```python
from build123d import *

# Parameters (mm, degrees)
SKETCH_1_R      = 7
SKETCH_1_R_2    = 4
EXTRUDE_1_DEPTH = 10
SKETCH_2_R      = 4
SKETCH_2_R_2    = 2.2
EXTRUDE_2_DEPTH = 7
CHAMFER_1_SIZE  = 1
CHAMFER_2_SIZE  = 0.5
CHAMFER_3_SIZE  = 0.5


with BuildPart() as part:
    # 草图1 → 凸台-拉伸1 (new body)
    with BuildSketch(Plane.XY):
        with Locations((42.877900702, -281.152618372)):
            Circle(SKETCH_1_R)
        with Locations((42.877900702, -281.152618372)):
            Circle(SKETCH_1_R_2, mode=Mode.SUBTRACT)
    extrude(amount=EXTRUDE_1_DEPTH)

    # 草图2 → 凸台-拉伸2 (add)
    with BuildSketch(Plane.XY.offset(-3)):
        with Locations((42.877900702, -281.152618372)):
            Circle(SKETCH_2_R)
        with Locations((42.877900702, -281.152618372)):
            Circle(SKETCH_2_R_2, mode=Mode.SUBTRACT)
    extrude(amount=EXTRUDE_2_DEPTH)

    # 倒角1
    chamfer_1_edges = [part.edges().sort_by_distance(p)[0] for p in [
        (35.877900702, -281.152618372, 0),
        (35.877900702, -281.152618372, 10),
    ]]
    chamfer(chamfer_1_edges, length=CHAMFER_1_SIZE)

    # 倒角2
    chamfer_2_edges = [part.edges().sort_by_distance(p)[0] for p in [
        (38.877900702, -281.152618372, -3),
    ]]
    chamfer(chamfer_2_edges, length=CHAMFER_2_SIZE)

    # 倒角3
    chamfer_3_edges = [part.edges().sort_by_distance(p)[0] for p in [
        (38.877900702, -281.152618372, 10),
    ]]
    chamfer(chamfer_3_edges, length=CHAMFER_3_SIZE)


solid = part.part
```
Work out the finished part from the listing and answer in its coordinate system (mm). A direction names the side the tool comes from. Coordinates: 2 decimals unless noted, no trailing zeros. Write each loop counter-clockwise with the first axis right and the second up, starting at its lowest first coordinate (ties: lowest second). Pieces come first, ordered by that corner, then holes.
Q1. Find the intervals of material crossed by line 1 (X direction, y = -281.75, z = 7.25); line 2 (X direction, y = -280.5, z = -2); line 3 (Y direction, x = 43.75, z = 5.5), in increasing order.
Q2. A cutting plane is placed at A-A, the plane z = 3.25. Give the vertices of the cut face in (x, y).
Q3. Each of these flat-tipped pins is pushed along its axis until it touches: pin 1 Ø2 at (x, z) = (44.5, 7.5) entering from -Y; pin 2 Ø4 at (x, y) = (42.88, -281.15) entering from +Z; pin 3 Ø1.5 at (y, z) = (-286, 6) entering from -X; pin 4 Ø5 at (y, z) = (-278, 8) entering from +X. Where does it stop, or does it pass through?
Q4. Determine the mould class of faces 4 (the face through (41, -283, -3)), 5 (the face through (42.59, -278.97, 0.45)), 6 (the face through (45.03, -277.78, -1.27)) for opening direction Y: released by +Y, released by -Y, zero draft, split by the parting line, or undercut.
Q5. Which of the six approach directions +Z, -Z, +X, -X, +Y, -Y give full straight-line access (tool end or side, diameter ignored) to faces 1 (the face through (47, -282, 0)), 2 (the face through (45.03, -277.78, 6.71)), 3 (the face through (45, -277, 10))?
Q6. A cutting plane is placed at B-B, the plane z = 5.75. Give the vertices of the cut face in (x, y), then the cut area to 3 significant figures.
Findings below:
1. line 1: x = 35.9 to 38.92, 46.83 to 49.85
1. line 2: x = 38.93 to 40.78, 44.98 to 46.82
1. line 3: y = -288.1 to -285.06, -277.25 to -274.21
2. outline: circle Ø14 at (42.88, -281.15); hole circle Ø4.4 at (42.88, -281.15)
3. pin 1: stops at y = -288.12
3. pin 2: passes through
3. pin 3: stops at x = 37.2
3. pin 4: stops at x = 49.85
4. face 4: zero draft
4. face 5: undercut
4. face 6: split by the parting line
5. face 1: -Z
5. face 2: +Z
5. face 3: +Z, +X, -X, +Y, -Y
6. outline: circle Ø14 at (42.88, -281.15); hole circle Ø8 at (42.88, -281.15)
6. area: 104 mm2
